Verification items for the finished model (mm, model axes). A direction names the side the tool comes from. Coordinates: 2 decimals unless noted, no trailing zeros. Write each loop counter-clockwise with the first axis right and the second up, starting at its lowest first coordinate (ties: lowest second). Pieces come first, ordered by that corner, then holes. Notation, with made-up numbers: (-13, 35) -> (43, 35) arc R11 ccw to (43, 52) -> close; hole circle Ø2 at (59.5, 7). An arc over 180 degrees is marked (long way). Answer in a Markdown table with one row per item.
```python
from build123d import *

# Parameters (mm, degrees)
SKETCH1_W           = 50.8
SKETCH1_H           = 25.4
SKETCH1_R           = 2.413
BOSS_EXTRUDE1_DEPTH = 1.143


with BuildPart() as part:
    # Sketch1 → Boss-Extrude1 (new, symmetric)
    with BuildSketch(Plane.XY):
        Rectangle(SKETCH1_W, SKETCH1_H)
        with Locations((-12.7, 0)):
            Circle(SKETCH1_R, mode=Mode.SUBTRACT)
        with Locations((12.7, 0)):
            Circle(SKETCH1_R, mode=Mode.SUBTRACT)
        Polygon((0, 7.62), (-6.599113577, 3.81), (-6.599113577, -3.81), (0, -7.62), (6.599113577, -3.81), (6.599113577, 3.81), align=None, mode=Mode.SUBTRACT)
    extrude(amount=BOSS_EXTRUDE1_DEPTH, both=True)


solid = part.part
```
1. Sectioned sample at C-C, the plane y = 6. Record the cut outline in (x, z).
Findings below:
| item | result |
|---|---|
| outline | (-25.4, -1.14) -> (-2.81, -1.14) -> (-2.81, 1.14) -> (-25.4, 1.14) -> close; (2.81, -1.14) -> (25.4, -1.14) -> (25.4, 1.14) -> (2.81, 1.14) -> close |
2. Sectioned sample at B-B, the plane y = 0. Record the cut outline in (x, z), and give its area (3 significant figures).
Findings below:
| item | result |
|---|---|
| outline | (-25.4, -1.14) -> (-15.11, -1.14) -> (-15.11, 1.14) -> (-25.4, 1.14) -> close; (-10.29, -1.14) -> (-6.6, -1.14) -> (-6.6, 1.14) -> (-10.29, 1.14) -> close; (6.6, -1.14) -> (10.29, -1.14) -> (10.29, 1.14) -> (6.6, 1.14) -> close; (15.11, -1.14) -> (25.4, -1.14) -> (25.4, 1.14) -> (15.11, 1.14) -> close |
| area | 63.9 mm² |
3. Release check for a two-part mould opening along Y. For faces 1 (the face through (25.4, 0, 0)), 2 (the face through (-3.346, -5.688, 0.016)), 3 (the face through (0, 12.7, 0)) record: released by +Y, released by -Y, zero draft, split by the parting line, or undercut.
Findings below:
| item | result |
|---|---|
| face 1 | zero draft |
| face 2 | undercut |
| face 3 | released by +Y |
4. Access from +Z, -Z, +X, -X, +Y, -Y to the whole of each face (thin tool, end or side, straight path). Record for faces 4 (the face through (5, -5, -1.143)), 5 (the face through (-6.599, 0, 0)).
Findings below:
| item | result |
|---|---|
| face 4 | -Z, +X, -X, +Y, -Y |
| face 5 | +Z, -Z |
5. Material ranges on probe 1 along Y at (x, z) = (12.7, 0.25); probe 2 along X at (y, z) = (-3.75, 0.6); probe 3 along Y at (x, z) = (-2, 0.5), recorded low to high. Write a range as from..to.
Findings below:
| item | result |
|---|---|
| probe 1 | y = -12.7..-2.41, 2.41..12.7 |
| probe 2 | x = -25.4..-6.6, 6.6..25.4 |
| probe 3 | y = -12.7..-6.47, 6.47..12.7 |
6. Sectioned sample at A-A, the plane x = 12.7. Record the cut outline in (y, z), and give its area (3 significant figures).
Findings below:
| item | result |
|---|---|
| outline | (-12.7, -1.14) -> (-2.41, -1.14) -> (-2.41, 1.14) -> (-12.7, 1.14) -> close; (2.41, -1.14) -> (12.7, -1.14) -> (12.7, 1.14) -> (2.41, 1.14) -> close |
| area | 47.0 mm² |
